from build123d import *

# Parameters (mm, degrees)
BOSS_EXTRUDE1_DEPTH     = 3
CUT_EXTRUDE4_DEPTH      = 62.713223867
CUT_EXTRUDE4_DEPTH_BACK = 62.713223867
SKETCH2_R               = 1.6
CUT_EXTRUDE8_DEPTH      = 1.55


with BuildPart() as part:
    # Sketch1 → Boss-Extrude1 (new body)
    with BuildSketch(Plane(origin=(0, 0, 0), x_dir=(1, 0, 0), z_dir=(0, 1, 0))):
        with BuildLine():
            Line((-3.3, -0.3), (-3.3, 48.56))
            ThreePointArc((-3.3, 48.56), (-2.421320344, 50.681320344), (-0.3, 51.56))
            Line((-0.3, 51.56), (30.78, 51.56))
            ThreePointArc((30.78, 51.56), (32.901320344, 50.681320344), (33.78, 48.56))
            Line((33.78, 48.56), (33.78, -0.3))
            ThreePointArc((33.78, -0.3), (32.901320344, -2.421320344), (30.78, -3.3))
            Line((30.78, -3.3), (-0.3, -3.3))
            ThreePointArc((-0.3, -3.3), (-2.421320344, -2.421320344), (-3.3, -0.3))
        make_face()
    extrude(amount=BOSS_EXTRUDE1_DEPTH)

    # Sketch2 → Cut-Extrude4 (cut, two sides: drawn at the far end of the back side and taken through both)
    with BuildSketch(Plane(origin=(0, 0, 0), x_dir=(1, 0, 0), z_dir=(0, 1, 0)).offset(-CUT_EXTRUDE4_DEPTH_BACK)):
        with Locations(Location((3.81, 43.18, 0), (0, 0, 270))):
            Circle(SKETCH2_R)
        with Locations(Location((26.67, 43.18, 0), (0, 0, 270))):
            Circle(SKETCH2_R)
        with Locations(Location((15.24, 3.81, 0), (0, 0, 270))):
            Circle(SKETCH2_R)
    extrude(amount=CUT_EXTRUDE4_DEPTH + CUT_EXTRUDE4_DEPTH_BACK, mode=Mode.SUBTRACT)

    # Sketch10 → Cut-Extrude8 (cut)
    with BuildSketch(Plane(origin=(0, 0, 0), x_dir=(-1, 0, 0), z_dir=(0, -1, 0))):
        Polygon((-1.21, 44.6811107), (-3.81, 46.1822214), (-6.41, 44.6811107), (-6.41, 41.6788893), (-3.81, 40.1777786), (-1.21, 41.6788893), align=None)
        Polygon((-24.07, 44.6811107), (-26.67, 46.1822214), (-29.27, 44.6811107), (-29.27, 41.6788893), (-26.67, 40.1777786), (-24.07, 41.6788893), align=None)
        Polygon((-12.64, 5.3111107), (-15.24, 6.8122214), (-17.84, 5.3111107), (-17.84, 2.3088893), (-15.24, 0.8077786), (-12.64, 2.3088893), align=None)
    extrude(amount=-CUT_EXTRUDE8_DEPTH, mode=Mode.SUBTRACT)


solid = part.part
Could you check a few things on this model? Use its own coordinates, in mm. A direction names the side the tool comes from. Round coordinates to 2 decimals unless told otherwise and drop trailing zeros. Write each loop counter-clockwise with the first axis right and the second up, starting at its lowest first coordinate (ties: lowest second). Pieces come first, ordered by that corner, then holes. Notation, with made-up numbers: (-7, 20.25) - (41, 20.25) arc R9 ccw to (41, 34.25) - close; hole circle Ø10 at (14.25, 55). An arc over 180 degrees is marked (long way). Put each result on its own line as item: value. Start each with the question number.
(1) Will this pin go through, and if not, where does the flat tip stop? pin 1 (1.6 mm diameter, centred on x = 3, z = -44, fed in from -Y).
(2) For faces 5 (the cylindrical face through (32.92, 1.48, 2.4)), 6 (the flat face through (12.64, 1, -4)), which set-ups out of +Z, -Z, +X, -X, +Y, -Y let a thin tool reach every point of the face, with its end or its side?
(3) Thinking about a two-plate mould opening in Z: for faces 1 (the flat face through (5.092, 0.764, -45.442)), 2 (the flat face through (15, 0, -25)), 3 (the flat face through (15, 1, 3.3)), 4 (the flat face through (5, 1.55, -41.89)), which applies, released by +Z, released by -Z, zero draft, split by the parting line, or undercut?
(4) I want a section at D-D, the plane x = 3. Please give me the cut outline in (y, z), plus the area to 3 significant figures.
(5) I want a section at C-C, the plane z = -43.18. Please give me the cut outline in (x, y), plus the area to 3 significant figures.
(6) I want a section at B-B, the plane z = -3.81. Please give me the cut outline in (x, y), plus the area to 3 significant figures.
(7) I need wall thicknesses on probe 1 along X at (y, z) = (1.95, -43.18); probe 2 along X at (y, z) = (1.3, -2.5); probe 3 along X at (y, z) = (1.9, -3.81). Which ranges of each line are inside material? Lowest first, please.
(8) I want a section at A-A, the plane y = 1. Please give me the cut outline in (x, z).
Here are the results:
1. pin 1: stops at y = 1.55
2. face 5: +Z, +X, +Y, -Y
2. face 6: -Y
3. face 1: undercut
3. face 2: zero draft
3. face 3: released by +Z
3. face 4: undercut
4. outline: (0, -51.56) - (3, -51.56) - (3, -44.56) - (1.55, -44.56) - (1.55, -45.71) - (0, -45.71) - close; (0, -40.65) - (1.55, -40.65) - (1.55, -41.8) - (3, -41.8) - (3, 3.3) - (0, 3.3) - close
4. area: 153 mm^2
5. outline: (-3.3, 0) - (1.21, 0) - (1.21, 1.55) - (2.21, 1.55) - (2.21, 3) - (-3.3, 3) - close; (5.41, 1.55) - (6.41, 1.55) - (6.41, 0) - (24.07, 0) - (24.07, 1.55) - (25.07, 1.55) - (25.07, 3) - (5.41, 3) - close; (28.27, 1.55) - (29.27, 1.55) - (29.27, 0) - (33.78, 0) - (33.78, 3) - (28.27, 3) - close
5. area: 85.8 mm^2
6. outline: (-3.3, 0) - (12.64, 0) - (12.64, 1.55) - (13.64, 1.55) - (13.64, 3) - (-3.3, 3) - close; (16.84, 1.55) - (17.84, 1.55) - (17.84, 0) - (33.78, 0) - (33.78, 3) - (16.84, 3) - close
6. area: 98.5 mm^2
7. probe 1: x = -3.3 to 2.21, 5.41 to 25.07, 28.27 to 33.78
7. probe 2: x = -3.3 to 12.64, 17.84 to 33.78
7. probe 3: x = -3.3 to 13.64, 16.84 to 33.78
8. outline: (-3.3, -48.56) arc R3 ccw to (-0.3, -51.56) - (30.78, -51.56) arc R3 ccw to (33.78, -48.56) - (33.78, 0.3) arc R3 ccw to (30.78, 3.3) - (-0.3, 3.3) arc R3 ccw to (-3.3, 0.3) - close; hole (1.21, -44.68) - (3.81, -46.18) - (6.41, -44.68) - (6.41, -41.68) - (3.81, -40.18) - (1.21, -41.68) - close; hole (12.64, -5.31) - (15.24, -6.81) - (17.84, -5.31) - (17.84, -2.31) - (15.24, -0.81) - (12.64, -2.31) - close; hole (24.07, -44.68) - (26.67, -46.18) - (29.27, -44.68) - (29.27, -41.68) - (26.67, -40.18) - (24.07, -41.68) - close
